The drawing under review shows one solid part. Ordinate dimensions are in mm from its lowest x, y, z. A direction names the side the tool comes from. Coordinates: 2 decimals unless noted, no trailing zeros. Loops run counter-clockwise (first coordinate to the right, second up) from the corner with the lowest first, then second, coordinate; pieces in that order, holes last. Notation, with made-up numbers: M -8,40 L 50,40 A31 ccw 50,78 Z; hole C -34,87 d8. An arc over 180 degrees is marked long. Use one line per item in the form item = value.
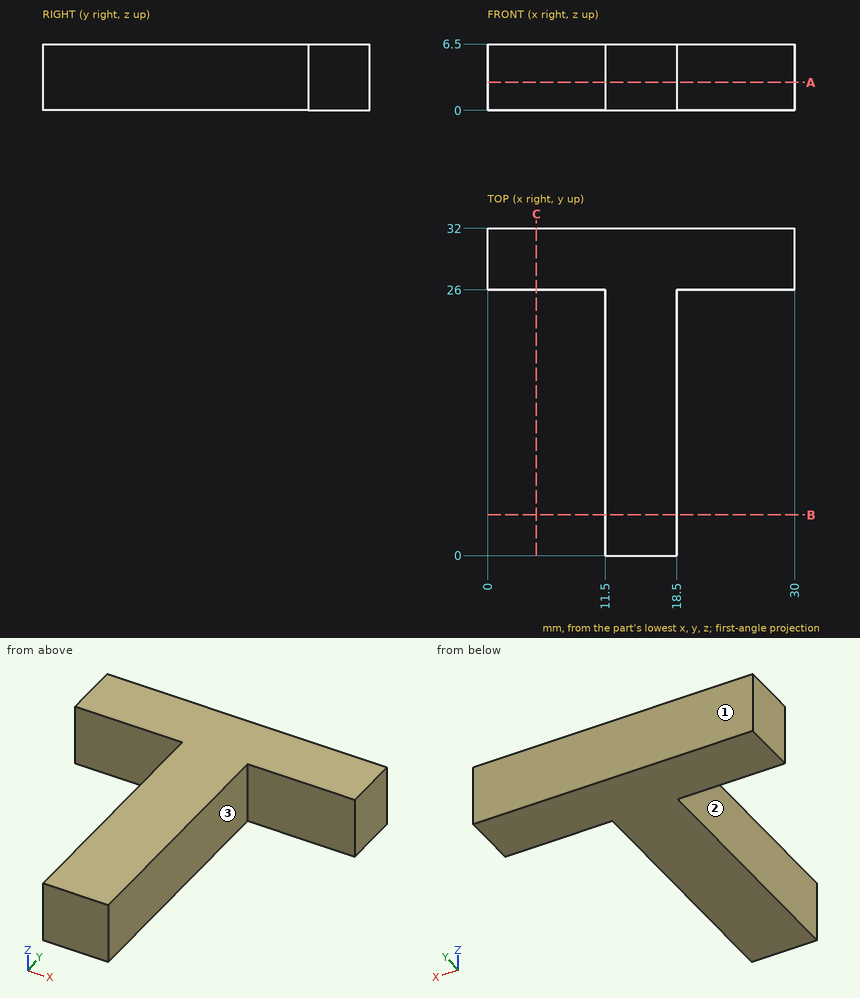
1. Consider section C-C on x = 4.75. Write out the cut boundary in (y, z), plus the area to 3 significant figures.
Computed values:
outline = M 26,0 L 32,0 L 32,6.5 L 26,6.5 Z
area = 39.0 mm2
2. For pin 1 Ø1.5 at (y, z) = (19, 1) entering from -X, flat-tipped, find the tip position at first contact; note if it passes through.
Computed values:
pin_1 = 11.5
3. Tool access review of the marked faces 1, 2 and 3: name each direction out of +Z, -Z, +X, -X, +Y, -Y from which nothing blocks a thin tool from reaching the whole face with its end or side.
Computed values:
face_1 = +Z, -Z, +X, -X, +Y
face_2 = +Z, -Z, -X, -Y
face_3 = +Z, -Z, +X, -Y
4. Consider section A-A on z = 2.75. Write out the cut boundary in (x, y), plus the area to 3 significant figures.
Computed values:
outline = M 0,26 L 11.5,26 L 11.5,0 L 18.5,0 L 18.5,26 L 30,26 L 30,32 L 0,32 Z
area = 362 mm2
5. Wall thickness on line 1 along Y through (x, z) = (21, 4.75); line 2 along X through (y, z) = (14, 2.5): over which ranges is each line inside the solid? List them lowest first. Write a range as from..to.
Computed values:
line_1 = 26..32
line_2 = 11.5..18.5
6. Consider section B-B on y = 4. Write out the cut boundary in (x, z), plus the area to 3 significant figures.
Computed values:
outline = M 11.5,0 L 18.5,0 L 18.5,6.5 L 11.5,6.5 Z
area = 45.5 mm2
